Build history of the part. All positions in model axes, mm. A direction names the side the tool comes from. Round coordinates to 2 decimals unless told otherwise and drop trailing zeros. Write each loop counter-clockwise with the first axis right and the second up, starting at its lowest first coordinate (ties: lowest second). Pieces come first, ordered by that corner, then holes. Notation, with made-up numbers: M 83,84.25 L 110,84.25 A12 ccw 110,101.25 Z; hole C 51,10.5 d3. An arc over 180 degrees is marked long. Use a Markdown table: item, result.
from build123d import *

# Parameters (mm, degrees)
SKETCH_1_W          = 125
SKETCH_1_H          = 25
SKETCH_1_R          = 1.45
SKETCH_1_R_2        = 1.95
EXTRUDE_1_DEPTH     = 3
CUT_EXTRUDE_1_DEPTH = 10
FILLET_1_R          = 2
FILLET_2_R          = 1


with BuildPart() as part:
    # 草图1 → 凸台-拉伸1 (new body)
    with BuildSketch(Plane.XY):
        with Locations((62.5, 12.5)):
            Rectangle(SKETCH_1_W, SKETCH_1_H)
        with Locations((32.5, 20)):
            Circle(SKETCH_1_R, mode=Mode.SUBTRACT)
        with Locations((57.5, 20)):
            Circle(SKETCH_1_R, mode=Mode.SUBTRACT)
        with Locations((57.5, 5)):
            Circle(SKETCH_1_R, mode=Mode.SUBTRACT)
        with Locations((32.5, 5)):
            Circle(SKETCH_1_R, mode=Mode.SUBTRACT)
        with Locations((5, 20)):
            Circle(SKETCH_1_R_2, mode=Mode.SUBTRACT)
        with Locations((5, 5)):
            Circle(SKETCH_1_R_2, mode=Mode.SUBTRACT)
        with Locations((120, 20)):
            Circle(SKETCH_1_R_2, mode=Mode.SUBTRACT)
        with Locations((120, 5)):
            Circle(SKETCH_1_R_2, mode=Mode.SUBTRACT)
    extrude(amount=EXTRUDE_1_DEPTH)

    # 草图2 → 切除-拉伸1 (cut)
    with BuildSketch(Plane.XY.offset(3)):
        Polygon((60.767753727, 21), (116, 21), (116, 9.114458974), align=None)
        Polygon((61.5, 15.727967439), (61.5, 4), (116, 4), align=None)
        Polygon((36.02221675, 21), (53.5, 21), (53.5, 11.425425105), align=None)
        Polygon((36.5, 16.432325355), (36.5, 4), (53.904028142, 4), align=None)
        Polygon((29.180055305, 21), (9, 21), (9, 7.144539038), align=None)
        Polygon((28.5, 15.183615903), (28.5, 2.402022244), (8.239478793, 2.402022244), align=None)
    extrude(amount=-CUT_EXTRUDE_1_DEPTH, mode=Mode.SUBTRACT)

    # 圆角1
    fillet_1_edges = [part.edges().sort_by_distance(p)[0] for p in [
        (0, 25, 1.5),
        (125, 25, 1.5),
        (125, 0, 1.5),
        (0, 0, 1.5),
    ]]
    fillet(fillet_1_edges, radius=FILLET_1_R)

    # 圆角2
    fillet_2_edges = [part.edges().sort_by_distance(p)[0] for p in [
        (116, 9.114458974, 1.5),
        (60.767753727, 21, 1.5),
        (116, 21, 1.5),
        (29.180055305, 21, 1.5),
        (9, 7.144539038, 1.5),
        (9, 21, 1.5),
        (36.5, 16.432325355, 1.5),
        (53.904028142, 4, 1.5),
        (36.5, 4, 1.5),
        (53.5, 11.425425105, 1.5),
        (36.02221675, 21, 1.5),
        (53.5, 21, 1.5),
        (61.5, 15.727967439, 1.5),
        (116, 4, 1.5),
        (61.5, 4, 1.5),
        (8.239478793, 2.402022244, 1.5),
        (28.5, 15.183615903, 1.5),
        (28.5, 2.402022244, 1.5),
    ]]
    fillet(fillet_2_edges, radius=FILLET_2_R)


solid = part.part
Q1. Cut at A-A on x = 57.5. Give the cut face in (y, z).
Response values:
| item | result |
|---|---|
| outline | M 0,0 L 3.55,0 L 3.55,3 L 0,3 Z; M 6.45,0 L 18.55,0 L 18.55,3 L 6.45,3 Z; M 21.45,0 L 25,0 L 25,3 L 21.45,3 Z |
Q2. Cut at C-C on x = 120. Give the cut face in (y, z), and give its area (3 significant figures).
Response values:
| item | result |
|---|---|
| outline | M 0,0 L 3.05,0 L 3.05,3 L 0,3 Z; M 6.95,0 L 18.05,0 L 18.05,3 L 6.95,3 Z; M 21.95,0 L 25,0 L 25,3 L 21.95,3 Z |
| area | 51.6 mm2 |
Q3. Drill centre lines: L1, parallel to Y at x = 5, z = 0.75; L2, parallel to Y at x = 57.5, z = 1.1; L3, parallel to Y at x = 67, z = 2.15. Where is each one in solid material? Low to high.
Response values:
| item | result |
|---|---|
| L1 | y = 0 to 3.05, 6.95 to 18.05, 21.95 to 25 |
| L2 | y = 0 to 3.55, 6.45 to 18.55, 21.45 to 25 |
| L3 | y = 0 to 4, 14.54 to 25 |
Q4. Which spindle directions (+Z, -Z, +X, -X, +Y, -Y) get a long thin tool onto all of the face, cutting with end or side? Do faces 1 (the cylindrical face through (69.172, 20.085, 1.479)), 2 (the cylindrical face through (124.4, 0.57, 1.52)). Say none if no direction does.
Response values:
| item | result |
|---|---|
| face 1 | +Z, -Z |
| face 2 | +Z, -Z, +X, -Y |
Q5. Cut at B-B on z = 1.9. Count the separate pieces of the cut face and the enclosed holes in it, and give its area (3 significant figures).
Response values:
| item | result |
|---|---|
| separate pieces | 1 |
| enclosed holes | 14 |
| area | 1,970 mm2 |
Q6. Two-plate mould, pull along X, no slides. Class faces 3 (the flat face through (45.822, 15.631, 1.521)), 4 (the flat face through (62, 0, 1)), 5 (the cylindrical face through (33.839, 19.445, 1.479)), 6 (the flat face through (125, 12, 1)): +X half, -X half, draft (parallel to the pull), parting line (faces both ways), or undercut.
Response values:
| item | result |
|---|---|
| face 3 | undercut |
| face 4 | draft |
| face 5 | undercut |
| face 6 | +X half |
